Input: part model. Units: mm. Frame: model coordinates. Face numbers are marked on the shaded views. A direction names the side the tool comes from. Round coordinates to 2 decimals unless told otherwise and drop trailing zeros. Loops run counter-clockwise (first coordinate to the right, second up) from the corner with the lowest first, then second, coordinate; pieces in that order, holes last. Notation, with made-up numbers: (-16, -0.75) -> (37, -0.75) arc R20 ccw to (37, 8.25) -> close; hole circle Ø8 at (-21, -8.5). An arc over 180 degrees is marked (long way). Answer in a Markdown table with one row per item. Add a question column.
Q1. Ray query, L1, parallel to Y at x = 1, z = -26; L2, parallel to X at y = -25.5, z = -9; L3, parallel to Z at x = 9.5, y = -25.5. Return the intervals inside material, ascending. Write a range as from..to.
Q2. Section B-B, the plane x = 6. Give the number of separate pieces and of enclosed holes in the cut face, and give its area (3 significant figures).
Q3. Reachability of the marked faces 1, 2 and 3 from +Z, -Z, +X, -X, +Y, -Y: full face, straight path, thin tool, end or side. Return the list, or none.
Q4. Mould query, pull axis Y, two halves, no side actions, for the marked faces 4, 5 and 6. Classes: pulls with the +Y half, pulls with the -Y half, needs draft (parallel to the pull), parting line crosses it, or undercut.
Q5. Pin query (flat end, axial travel): pin 1 (2 mm diameter, centred on x = 9, z = -0.5, fed in from -Y); pin 2 (2 mm diameter, centred on y = 7.5, z = -5.5, fed in from +X); pin 3 (3 mm diameter, centred on x = 17, y = -22, fed in from -Z). Return the tip coordinate at first contact, or that it passes through.
Q6. Section A-A, the plane z = 0. Output: boundary loops of the cut face in (x, y), and give its area (3 significant figures).
```python
from build123d import *

# Parameters (mm, degrees)
SKETCH1_R                 = 36
SKETCH1_R_2               = 1.075
SKETCH1_R_3               = 4.25
BOSS_EXTRUDE1_DEPTH       = 3
SKETCH1_3_R               = 4.25
BOSS_EXTRUDE2_DEPTH       = 20
BOSS_EXTRUDE3_DEPTH       = 3
BOSS_EXTRUDE5_DEPTH       = 17
SKETCH3_R                 = 2.2
CUT_EXTRUDE1_DEPTH        = 10
BOSS_EXTRUDE6_DEPTH       = 17
CUT_EXTRUDE2_START        = 3
CUT_EXTRUDE2_DEPTH        = 17
BOSS_EXTRUDE7_START       = 3
BOSS_EXTRUDE7_OUTLINE_R   = 2.1
BOSS_EXTRUDE7_OUTLINE_R_2 = 0.1
BOSS_EXTRUDE7_DEPTH       = 14
FILLET1_R                 = 0.5


# Read off the part's stored shape, not the designer's step: Cut-Extrude2, Boss-Extrude7
with BuildPart() as part:
    # Sketch1 → Boss-Extrude1 (new body)
    with BuildSketch(Plane(origin=(0, 0, 0), x_dir=(0, 0, -1), z_dir=(1, 0, 0))):
        Circle(SKETCH1_R)
        with Locations((20.089039043, 27.430466826)):
            Circle(SKETCH1_R_2, mode=Mode.SUBTRACT)
        with Locations((23.711117025, 24.36766155)):
            Circle(SKETCH1_R_2, mode=Mode.SUBTRACT)
        with Locations((26.871685085, 20.830567459)):
            Circle(SKETCH1_R_2, mode=Mode.SUBTRACT)
        with Locations((29.509226361, 16.888030067)):
            Circle(SKETCH1_R_2, mode=Mode.SUBTRACT)
        with Locations((31.572404113, 12.61678638)):
            Circle(SKETCH1_R_2, mode=Mode.SUBTRACT)
        with Locations((33.021060931, 8.099971297)):
            Circle(SKETCH1_R_2, mode=Mode.SUBTRACT)
        with Locations((33.827000359, 3.425499486)):
            Circle(SKETCH1_R_2, mode=Mode.SUBTRACT)
        with Locations((33.974535702, -1.315645775)):
            Circle(SKETCH1_R_2, mode=Mode.SUBTRACT)
        with Locations((33.460795354, -6.031183488)):
            Circle(SKETCH1_R_2, mode=Mode.SUBTRACT)
        with Locations((32.295778685, -10.629331075)):
            Circle(SKETCH1_R_2, mode=Mode.SUBTRACT)
        with Locations((30.50216142, -15.020590824)):
            Circle(SKETCH1_R_2, mode=Mode.SUBTRACT)
        with Locations((28.114854279, -19.119491857)):
            Circle(SKETCH1_R_2, mode=Mode.SUBTRACT)
        with Locations((25.180323479, -22.84625373)):
            Circle(SKETCH1_R_2, mode=Mode.SUBTRACT)
        with Locations((21.755686325, -26.128339261)):
            Circle(SKETCH1_R_2, mode=Mode.SUBTRACT)
        with Locations((17.907599484, -28.901866388)):
            Circle(SKETCH1_R_2, mode=Mode.SUBTRACT)
        with Locations((13.710961588, -31.112851562)):
            Circle(SKETCH1_R_2, mode=Mode.SUBTRACT)
        with Locations((9.24745542, -32.718260471)):
            Circle(SKETCH1_R_2, mode=Mode.SUBTRACT)
        with Locations((4.603958052, -33.686845656)):
            Circle(SKETCH1_R_2, mode=Mode.SUBTRACT)
        with Locations((-0.129150123, -33.999754709)):
            Circle(SKETCH1_R_2, mode=Mode.SUBTRACT)
        with Locations((-4.859744537, -33.65089721)):
            Circle(SKETCH1_R_2, mode=Mode.SUBTRACT)
        with Locations((-9.495749552, -32.647063274)):
            Circle(SKETCH1_R_2, mode=Mode.SUBTRACT)
        with Locations((-13.946930604, -31.007791388)):
            Circle(SKETCH1_R_2, mode=Mode.SUBTRACT)
        with Locations((-18.126650515, -28.764988112)):
            Circle(SKETCH1_R_2, mode=Mode.SUBTRACT)
        with Locations((-21.953555793, -25.962307063)):
            Circle(SKETCH1_R_2, mode=Mode.SUBTRACT)
        with Locations((-25.353160079, -22.654299239)):
            Circle(SKETCH1_R_2, mode=Mode.SUBTRACT)
        with Locations((-28.259293943, -18.905351249)):
            Circle(SKETCH1_R_2, mode=Mode.SUBTRACT)
        with Locations((-30.615392795, -14.788432101)):
            Circle(SKETCH1_R_2, mode=Mode.SUBTRACT)
        with Locations((-32.375597851, -10.383672944)):
            Circle(SKETCH1_R_2, mode=Mode.SUBTRACT)
        with Locations((-33.505648721, -5.776807404)):
            Circle(SKETCH1_R_2, mode=Mode.SUBTRACT)
        with Locations((-33.983550251, -1.057502879)):
            Circle(SKETCH1_R_2, mode=Mode.SUBTRACT)
        with Locations((-33.800000631, 3.682384736)):
            Circle(SKETCH1_R_2, mode=Mode.SUBTRACT)
        with Locations((-32.958572446, 8.350598921)):
            Circle(SKETCH1_R_2, mode=Mode.SUBTRACT)
        with Locations((-31.475643138, 12.856278197)):
            Circle(SKETCH1_R_2, mode=Mode.SUBTRACT)
        with Locations((-29.380076239, 17.111724641)):
            Circle(SKETCH1_R_2, mode=Mode.SUBTRACT)
        with Locations((-26.712659575, 21.03411083)):
            Circle(SKETCH1_R_2, mode=Mode.SUBTRACT)
        with Locations((-23.525311378, 24.547091977)):
            Circle(SKETCH1_R_2, mode=Mode.SUBTRACT)
        with Locations((-19.880069755, 27.582291901)):
            Circle(SKETCH1_R_2, mode=Mode.SUBTRACT)
        with Locations((-15.847885187, 30.080633888)):
            Circle(SKETCH1_R_2, mode=Mode.SUBTRACT)
        with Locations((-11.507239561, 31.993490552)):
            Circle(SKETCH1_R_2, mode=Mode.SUBTRACT)
        with Locations((-6.942618606, 33.283630314)):
            Circle(SKETCH1_R_2, mode=Mode.SUBTRACT)
        with Locations((-2.242867477, 33.925942072)):
            Circle(SKETCH1_R_2, mode=Mode.SUBTRACT)
        with Locations((2.500538516, 33.907923958)):
            Circle(SKETCH1_R_2, mode=Mode.SUBTRACT)
        with Locations((7.195274371, 33.229926673)):
            Circle(SKETCH1_R_2, mode=Mode.SUBTRACT)
        with Locations((11.749962396, 31.905146665)):
            Circle(SKETCH1_R_2, mode=Mode.SUBTRACT)
        with Locations((16.075950767, 29.959369268)):
            Circle(SKETCH1_R_2, mode=Mode.SUBTRACT)
        Circle(SKETCH1_R_3, mode=Mode.SUBTRACT)
    extrude(amount=BOSS_EXTRUDE1_DEPTH)

    # Sketch1<3> → Boss-Extrude2 (add)
    with BuildSketch(Plane(origin=(0, 0, 0), x_dir=(0, 0, -1), z_dir=(1, 0, 0))):
        Circle(SKETCH1_3_R)
        with BuildLine():
            ThreePointArc((2.05, -1.55), (2.570019455, 0), (2.05, 1.55))
            Line((2.05, 1.55), (-2.05, 1.55))
            ThreePointArc((-2.05, 1.55), (-2.570019455, 0), (-2.05, -1.55))
            Line((-2.05, -1.55), (2.05, -1.55))
        make_face(mode=Mode.SUBTRACT)
    extrude(amount=BOSS_EXTRUDE2_DEPTH)

    # Sketch1<4> → Boss-Extrude3 (add)
    with BuildSketch(Plane(origin=(0, 0, 0), x_dir=(0, 0, -1), z_dir=(1, 0, 0))):
        with BuildLine():
            Line((-2.05, -1.55), (2.05, -1.55))
            ThreePointArc((2.05, -1.55), (2.570019455, 0), (2.05, 1.55))
            Line((2.05, 1.55), (-2.05, 1.55))
            ThreePointArc((-2.05, 1.55), (-2.570019455, 0), (-2.05, -1.55))
        make_face()
    extrude(amount=BOSS_EXTRUDE3_DEPTH)

    # Sketch2 → Boss-Extrude5 (add)
    with BuildSketch(Plane(origin=(3, 0, 0), x_dir=(0, 0, -1), z_dir=(1, 0, 0))):
        with BuildLine():
            Line((-27.493123978, -9.984519716), (-3.619491149, -2.227506189))
            ThreePointArc((-3.619491149, -2.227506189), (-4.041990194, -1.313322226), (-4.237525138, -0.325393156))
            Line((-4.237525138, -0.325393156), (-28.111157966, -8.082406683))
            ThreePointArc((-28.111157966, -8.082406683), (-27.818403102, -9.038747085), (-27.493123978, -9.984519716))
        make_face()
        with BuildLine():
            ThreePointArc((1.618934563, 3.92957388), (2.498087322, 3.438322226), (3.236968552, 2.754003376))
            Line((3.236968552, 2.754003376), (17.991685075, 23.062128439))
            ThreePointArc((17.991685075, 23.062128439), (17.19271863, 23.663747085), (16.373651086, 24.237698944))
            Line((16.373651086, 24.237698944), (1.618934563, 3.92957388))
        make_face()
        with BuildLine():
            ThreePointArc((4.237525138, -0.325393156), (4.041990194, -1.313322226), (3.619491149, -2.227506189))
            Line((3.619491149, -2.227506189), (27.493123978, -9.984519716))
            ThreePointArc((27.493123978, -9.984519716), (27.818403102, -9.038747085), (28.111157966, -8.082406683))
            Line((28.111157966, -8.082406683), (4.237525138, -0.325393156))
        make_face()
        with BuildLine():
            ThreePointArc((1, -4.13067791), (0, -4.25), (-1, -4.13067791))
            Line((-1, -4.13067791), (-1, -29.232900985))
            ThreePointArc((-1, -29.232900985), (0, -29.25), (1, -29.232900985))
            Line((1, -29.232900985), (1, -4.13067791))
        make_face()
        with BuildLine():
            Line((-3.236968552, 2.754003376), (-17.991685075, 23.062128439))
            ThreePointArc((-17.991685075, 23.062128439), (-17.19271863, 23.663747085), (-16.373651086, 24.237698944))
            Line((-16.373651086, 24.237698944), (-1.618934563, 3.92957388))
            ThreePointArc((-1.618934563, 3.92957388), (-2.498087322, 3.438322226), (-3.236968552, 2.754003376))
        make_face()
    extrude(amount=BOSS_EXTRUDE5_DEPTH)

    # Sketch3 → Cut-Extrude1 (cut)
    with BuildSketch(Plane.ZY):
        Circle(SKETCH3_R)
    extrude(amount=-CUT_EXTRUDE1_DEPTH, mode=Mode.SUBTRACT)

    # Sketch6 → Boss-Extrude6 (add)
    with BuildSketch(Plane(origin=(3, 0, 0), x_dir=(0, 0, -1), z_dir=(1, 0, 0))):
        with BuildLine():
            ThreePointArc((9.977852523, 8.090169944), (9.530979272, 9.951530993), (8.287772057, 11.407139621))
            Line((8.287772057, 11.407139621), (7.112201553, 9.789105632))
            ThreePointArc((7.112201553, 9.789105632), (7.748966224, 9.043549993), (7.977852523, 8.090169944))
            ThreePointArc((7.977852523, 8.090169944), (6.831232572, 6.219056243), (4.643503493, 6.391234256))
            Line((4.643503493, 6.391234256), (3.467932989, 4.773200267))
            ThreePointArc((3.467932989, 4.773200267), (7.739213572, 4.437043195), (9.977852523, 8.090169944))
        make_face()
        with BuildLine():
            Line((7.112201553, 9.789105632), (8.287772057, 11.407139621))
            ThreePointArc((8.287772057, 11.407139621), (2.560882846, 10.500089478), (3.467932989, 4.773200267))
            Line((3.467932989, 4.773200267), (4.643503493, 6.391234256))
            ThreePointArc((4.643503493, 6.391234256), (4.178916835, 9.324518974), (7.112201553, 9.789105632))
        make_face()
    extrude(amount=BOSS_EXTRUDE6_DEPTH)

    # Cut-Extrude2 outline → Cut-Extrude2 (cut)
    with BuildSketch(Plane.YZ.offset(CUT_EXTRUDE2_START)):
        with BuildLine():
            Line((10.17190097, -6.154250668), (7.184009422, -3.983420389))
            ThreePointArc((7.184009422, -3.983420389), (6.391234256, -4.643503493), (6.008438918, -5.601454378))
            Line((6.008438918, -5.601454378), (8.996330465, -7.772284657))
            ThreePointArc((8.996330465, -7.772284657), (9.789105632, -7.112201553), (10.17190097, -6.154250668))
        make_face()
    extrude(amount=CUT_EXTRUDE2_DEPTH, mode=Mode.SUBTRACT)

    # Boss-Extrude7 outline → Boss-Extrude7 (add)
    with BuildSketch(Plane.YZ.offset(BOSS_EXTRUDE7_START)):
        with Locations((8.090169944, -5.877852523)):
            Circle(BOSS_EXTRUDE7_OUTLINE_R)
        with Locations((8.090169944, -5.877852523)):
            Circle(BOSS_EXTRUDE7_OUTLINE_R_2, mode=Mode.SUBTRACT)
    extrude(amount=BOSS_EXTRUDE7_DEPTH)

    # Fillet1
    fillet1_edges = [part.edges().sort_by_distance(p)[0] for p in [
        (20, 6.855820914, -7.576788211),
    ]]
    fillet(fillet1_edges, radius=FILLET1_R)


solid = part.part
```
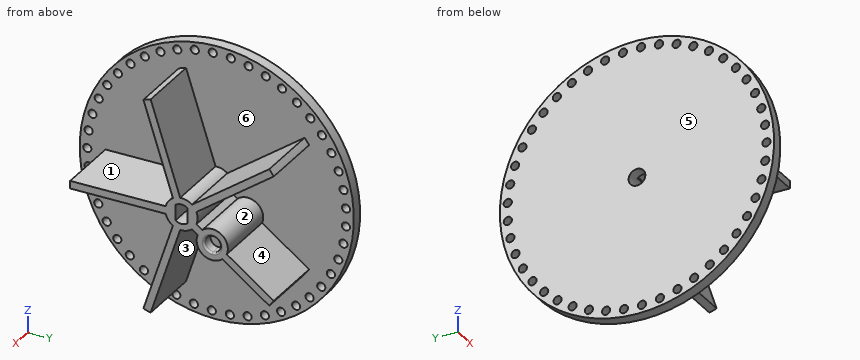
Answer block:
| question | item | result |
|---|---|---|
| 1 | L1 | -24.9..-23.54, -22.15..20.2, 21.46..24.9 |
| 1 | L2 | 0..3 |
| 1 | L3 | -1..1 |
| 2 | separate pieces | 1 |
| 2 | enclosed holes | 2 |
| 2 | area | 326 mm^2 |
| 3 | face 1 | +X, -Y |
| 3 | face 2 | +X |
| 3 | face 3 | -Z, +X |
| 4 | face 4 | pulls with the +Y half |
| 4 | face 5 | needs draft |
| 4 | face 6 | undercut |
| 5 | pin 1 | y = -29.25 |
| 5 | pin 2 | x = 17 |
| 5 | pin 3 | z = -1 |
| 6 | outline | (0, -36) -> (3, -36) -> (3, -35.07) -> (0, -35.07) -> close; (0, -32.93) -> (3, -32.93) -> (3, -29.25) -> (20, -29.25) -> (20, -1.55) -> (10, -1.55) -> (10, -2.2) -> (0, -2.2) -> close; (0, 2.2) -> (10, 2.2) -> (10, 1.55) -> (20, 1.55) -> (20, 4.25) -> (3, 4.25) -> (3, 36) -> (0, 36) -> close |
| 6 | area | 704 mm^2 |
